Design review of the part built by this model. Coordinates are the model's own, in mm. Face numbers are marked on the shaded views. A direction names the side the tool comes from. Give positions to 0.01 mm unless a question says otherwise; leave off trailing zeros. Order: outer loops, then holes, each group sorted by start corner. A loop starts at its lowest first (then second) coordinate and runs counter-clockwise, first axis right, second up. Notation, with made-up numbers: (64, 25) -> (95, 25) arc R30 cw to (95, 55) -> close; hole circle Ø8 at (24, 72). An arc over 180 degrees is marked (long way). One line per item, written item: value.
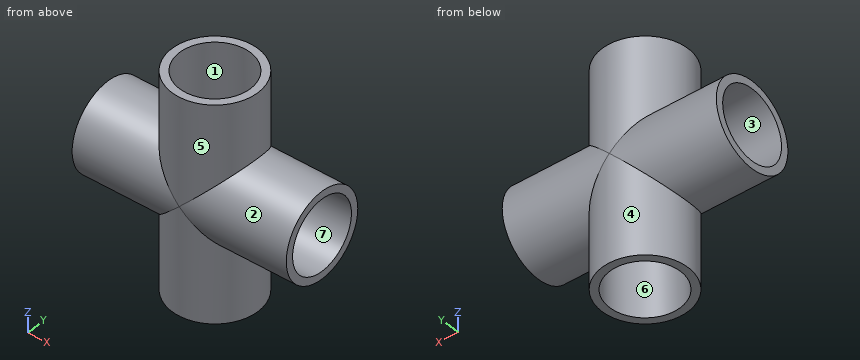
Autodesk Inventor part; units mm, degrees
ref_plane "Work Plane1" through (0, 0, 0) normal (-1, 0, 0) x (0, 1, 0)
ref_plane "YZ Plane" through (0, 0, 0) normal (1, 0, 0) x (0, 1, 0)
ref_plane "XZ Plane" through (0, 0, 0) normal (0, 1, 0) x (-1, 0, 0)
sketch "Sketch1" plane through (0, 0, 0) normal (0, 0, 1) x (1, 0, 0)
  circle A0 centre (0, 0) radius 20.3835
  dimension "d0" = 40.767
extrude "Extrusion1" add sketch "Sketch1" against normal blind 101.6
sketch "Sketch2" plane through (0, 0, 0) normal (0, 0, 1) x (1, 0, 0)
  line L0 (0, 0) -> (0, 19.704)
sketch "Sketch3" plane through (0, 0, -101.6) normal (0, 0, -1) x (-1, 0, 0)
  line L0 (0, 0) -> (0, 20.098)
ref_plane "Work Plane1" through (0, 0, 0) normal (-1, 0, 0) x (0, 1, 0)
sketch "Sketch4" plane through (0, 0, 0) normal (-1, 0, 0) x (0, 1, 0)
  circle A0 centre (0, 50.8) radius 20.3835
  point P0 (0, 0)
extrude "Extrusion2" add sketch "Sketch4" along normal mid plane 101.6
sketch "Sketch5" plane through (0, 0, 0) normal (0, 0, 1) x (1, 0, 0)
  circle A0 centre (0, 0) radius 16.7767
  dimension "d5" = 33.5534
sketch "Sketch6" plane through (50.8, 0, -50.8) normal (1, 0, 0) x (0, 0, -1)
  circle A0 centre (0, 0) radius 16.7767
  point P0 (-50.8, 0)
  dimension "d6" = 33.5534
sketch "Sketch7" plane through (0, 0, -101.6) normal (0, 0, -1) x (-1, 0, 0)
  circle A0 centre (0, 0) radius 20.3835
  circle A1 centre (0, 0) radius 16.7767
  dimension "d7" = 33.5534
sketch "Sketch8" plane through (-50.8, 0, -50.8) normal (-1, 0, 0) x (0, 0, 1)
  circle A0 centre (0, 0) radius 16.7767
  point P0 (50.8, 0)
  dimension "d8" = 33.5534
extrude "Extrusion3" cut sketch "Sketch5" against normal blind 31.75
extrude "Extrusion4" cut sketch "Sketch6" against normal blind 31.75
extrude "Extrusion5" cut sketch "Sketch7" against normal blind 31.75 contours A1
extrude "Extrusion6" cut sketch "Sketch8" against normal blind 31.75
sketch "Sketch9" plane through (0, 0, 0) normal (0, 0, 1) x (1, 0, 0)
  circle A0 centre (0, 0) radius 12.7
  dimension "d17" = 25.4
sketch "Sketch10" plane through (50.8, 0, -50.8) normal (1, 0, 0) x (0, 0, -1)
  circle A0 centre (0, 0) radius 12.7
  point P0 (-50.8, 0)
  dimension "d18" = 25.4
extrude "Extrusion7" cut sketch "Sketch10" against normal blind 101.6
extrude "Extrusion8" cut sketch "Sketch9" against normal blind 101.6
properties part number "Cross 1 Inch"
Item 1: Add section D-D on y = 0. Count the separate pieces of the cut face and the enclosed holes in it, plus the area to 3 significant figures.
Returned:
separate pieces: 4
enclosed holes: 0
area: 1,070 mm²
Item 2: Clearance check with flat-ended pins moving along their axes: P1, Ø8, axis at x = -36, y = 6, coming from the +Z side; P2, Ø6, axis at x = -9, z = -47, coming from the +Y side; P3, Ø5, axis at x = -37, z = -41, coming from the +Y side; P4, Ø10, axis at x = 22, y = 2, coming from the +Z side. State where each tip first meets the part, or that it passes through.
Returned:
P1: z = -30.51
P2: y = 20.37
P3: y = 19.03
P4: z = 0
Item 3: Draft analysis for pull direction X (two halves, no side actions). For the marked faces 5, 6 and 7, state which applies: pulls with the +X half, pulls with the -X half, needs draft (parallel to the pull), parting line crosses it, or undercut.
Returned:
face 5: parting line crosses it
face 6: undercut
face 7: needs draft
Item 4: Add section B-B on x = 5. Give the boundary of the cut face in (y, z).
Returned:
outline: (-19.76, -101.6) -> (-16.01, -101.6) -> (-16.01, -69.85) -> (-11.67, -69.85) -> (-11.67, -55.8) arc R12.7 cw to (-11.67, -45.8) -> (-11.67, -31.75) -> (-16.01, -31.75) -> (-16.01, 0) -> (-19.76, 0) -> (-19.76, -45.8) arc R20.38 ccw to (-19.76, -55.8) -> close; (11.67, -69.85) -> (16.01, -69.85) -> (16.01, -101.6) -> (19.76, -101.6) -> (19.76, -55.8) arc R20.38 ccw to (19.76, -45.8) -> (19.76, 0) -> (16.01, 0) -> (16.01, -31.75) -> (11.67, -31.75) -> (11.67, -45.8) arc R12.7 cw to (11.67, -55.8) -> close
Item 5: Add section A-A on z = -55. Give the boundary of the cut face in (x, y).
Returned:
outline: (-50.8, -19.95) -> (-4.2, -19.95) arc R20.38 ccw to (4.2, -19.95) -> (50.8, -19.95) -> (50.8, -16.24) -> (19.05, -16.24) -> (19.05, -11.99) -> (4.2, -11.99) arc R12.7 cw to (-4.2, -11.99) -> (-19.05, -11.99) -> (-19.05, -16.24) -> (-50.8, -16.24) -> close; (-50.8, 16.24) -> (-19.05, 16.24) -> (-19.05, 11.99) -> (-4.2, 11.99) arc R12.7 cw to (4.2, 11.99) -> (19.05, 11.99) -> (19.05, 16.24) -> (50.8, 16.24) -> (50.8, 19.95) -> (4.2, 19.95) arc R20.38 ccw to (-4.2, 19.95) -> (-50.8, 19.95) -> close
Item 6: To check wall thickness, follow line 1 along Y through (x, z) = (0, -40.5); line 2 along Z through (x, y) = (39, -10); line 3 along Y through (x, z) = (-10, -63). State the ranges of each line that lie inside material, in increasing order. Write a range as from..to.
Returned:
line 1: -20.38..-12.7, 12.7..20.38
line 2: -68.56..-64.27, -37.33..-33.04
line 3: -17.76..-7.83, 7.83..17.76
Item 7: Add section C-C on x = 34. Give the boundary of the cut face in (y, z).
Returned:
outline: circle Ø40.77 at (0, -50.8); hole circle Ø33.55 at (0, -50.8)
Item 8: Machinability: for the marked faces 1, 2, 3 and 4, which of the approach directions +Z, -Z, +X, -X, +Y, -Y give a long, thin tool a straight path to every point of the face, cutting with its end or side? Answer none if there is none.
Returned:
face 1: +Z
face 2: +X
face 3: -X
face 4: -Z
